Here's how the part is built. I have some questions about the finished solid (model axes, mm). A direction names the side the tool comes from. Give positions to 0.01 mm unless a question says otherwise; leave off trailing zeros. Loops run counter-clockwise (first coordinate to the right, second up) from the corner with the lowest first, then second, coordinate; pieces in that order, holes last.
Q1. Suppose I cut it at A-A (x = 0). List the corners of the cut face in (y, z) for me, and give its area (3 significant figures).
Q2. I'm going to push flat-ended pins straight in: P1, Ø6, axis at x = -2, y = 31.5, coming from the -Z side; P2, Ø3.5, axis at x = 1, y = 35.5, coming from the +Z side. Where does each tip first touch, or does it pass through?
Q3. Suppose I cut it at D-D (y = 11). List the corners of the cut face in (x, z) for me.
Q4. Suppose I cut it at C-C (z = 51.5). List the corners of the cut face in (x, y) for me.
Q5. For faces 4 (the face through (4, -4, 12.5)), 5 (the face through (0, 50, 35)), 6 (the face through (4, -4, 57.5)), which set-ups out of +Z, -Z, +X, -X, +Y, -Y let a thin tool reach every point of the face, with its end or its side?
Q6. Thinking about a two-plate mould opening in Z: for faces 1 (the face through (-1.08, -4.88, 6.16)), 2 (the face through (0, 0, 70)), 3 (the face through (0, 30, 17.5)), which applies, pulls with the +Z half, pulls with the -Z half, needs draft (parallel to the pull), parting line crosses it, or undercut?
Q7. I need wall thicknesses on probe 1 along Z at (x, y) = (-4.75, 47); probe 2 along Y at (x, z) = (-0.25, 19); probe 3 along Z at (x, y) = (4.75, 3). Which ranges of each line are inside material? Lowest first, please.
Q8. Suppose I cut it at B-B (y = 1.5). List the corners of the cut face in (x, z) for me, and give its area (3 significant figures).
```python
from build123d import *

# Parameters (mm, degrees)
SKETCH_1_R      = 5
EXTRUDE_1_DEPTH = 12.5
SKETCH_2_R      = 6
EXTRUDE_2_DEPTH = 22.5
SKETCH_3_R      = 5
EXTRUDE_3_DEPTH = 12.5
SKETCH_4_W      = 12
SKETCH_4_H      = 35
EXTRUDE_4_DEPTH = 50


with BuildPart() as part:
    # 草图1 → 凸台-拉伸1 (new body)
    with BuildSketch(Plane.XY):
        Circle(SKETCH_1_R)
    extrude(amount=EXTRUDE_1_DEPTH)

    # 草图2 → 凸台-拉伸2 (add)
    with BuildSketch(Plane.XY.offset(12.5)):
        with Locations(Location((0, 0, 0), (0, 0, 180))):
            Circle(SKETCH_2_R)
    extrude_2 = extrude(amount=EXTRUDE_2_DEPTH)

    # 镜向2: 凸台-拉伸2 across plane
    add(extrude_2.mirror(Plane.XY.offset(35)))

    # 草图3 → 凸台-拉伸3 (add)
    with BuildSketch(Plane.XY.offset(57.5)):
        Circle(SKETCH_3_R)
    extrude(amount=EXTRUDE_3_DEPTH)

    # 草图4 → 凸台-拉伸4 (add)
    with BuildSketch(Plane(origin=(0, 0, 0), x_dir=(1, 0, 0), z_dir=(0, 1, 0))):
        with Locations((0, -35)):
            Rectangle(SKETCH_4_W, SKETCH_4_H)
    extrude(amount=EXTRUDE_4_DEPTH)


solid = part.part
```
Solutions:
1. outline: (-6, 12.5) - (-5, 12.5) - (-5, 0) - (5, 0) - (5, 12.5) - (6, 12.5) - (6, 17.5) - (50, 17.5) - (50, 52.5) - (6, 52.5) - (6, 57.5) - (5, 57.5) - (5, 70) - (-5, 70) - (-5, 57.5) - (-6, 57.5) - close
1. area: 2,330 mm2
2. P1: stops at z = 17.5
2. P2: stops at z = 52.5
3. outline: (-6, 17.5) - (6, 17.5) - (6, 52.5) - (-6, 52.5) - close
4. outline: (-6, 0) arc R6 ccw to (6, 0) - (6, 50) - (-6, 50) - close
5. face 4: -Z
5. face 5: +Z, -Z, +X, -X, +Y
5. face 6: +Z
6. face 1: needs draft
6. face 2: pulls with the +Z half
6. face 3: pulls with the -Z half
7. probe 1: z = 17.5 to 52.5
7. probe 2: y = -5.99 to 50
7. probe 3: z = 12.5 to 57.5
8. outline: (-6, 17.5) - (-5.81, 17.5) - (-5.81, 12.5) - (-4.77, 12.5) - (-4.77, 0) - (4.77, 0) - (4.77, 12.5) - (5.81, 12.5) - (5.81, 17.5) - (6, 17.5) - (6, 52.5) - (5.81, 52.5) - (5.81, 57.5) - (4.77, 57.5) - (4.77, 70) - (-4.77, 70) - (-4.77, 57.5) - (-5.81, 57.5) - (-5.81, 52.5) - (-6, 52.5) - close
8. area: 775 mm2
